Part model, mm, in its own coordinate system. A direction names the side the tool comes from. Round coordinates to 2 decimals unless told otherwise and drop trailing zeros. Loops run counter-clockwise (first coordinate to the right, second up) from the corner with the lowest first, then second, coordinate; pieces in that order, holes last.
Solid Edge part; units mm, degrees
sketch "Sketch1" plane through (0, 0, 0) normal (0, -1, 0) x (1, 0, 0)
  line L0 (-51.028, 6) -> (118.972, 6)
  line L1 (118.972, 6) -> (118.972, -6)
  line L2 (118.972, -6) -> (-51.028, -6)
  line L3 (-51.028, -6) -> (-51.028, 6)
extrude "Protrusion1" add sketch "Sketch1" against normal blind 200
sketch "Sketch2" plane through (33.972, 100, 6) normal (0, 0, 1) x (0, 1, 0)
  line L0 (-100, -85) -> (100, 0)
extrude "ExtrudedCutout_3" cut sketch "Sketch2" against normal blind 139.4118 material side at (76.518, 100.0196, 6)
sketch "Sketch3" plane through (33.972, 0, 0) normal (0, -1, 0) x (1, 0, 0)
  line L0 (-73.94, 3) -> (-73.94, -3)
  line L1 (-73.94, -3) -> (-78.94, 0)
  line L2 (-78.94, 0) -> (-73.94, 3)
extrude "ExtrudedCutout_4" cut sketch "Sketch3" against normal blind 2.5
sketch "Sketch4" plane through (-42.468, 2.5, 0) normal (0, -1, 0) x (0.8574929, 0, -0.5144958)
  circle A0 centre (0, 0) radius 1.25
extrude "ExtrudedCutout_5" cut sketch "Sketch4" against normal blind 2.5
chamfer "Chamfer_6" distance 12 angle 45 2 edges at (76.472, 100, 6) (76.472, 100, -6)
chamfer "Chamfer_7" distance 12 angle 45 2 edges at (-15.0474, 200, 6) (-15.0474, 200, -6)
chamfer "Chamfer_8" distance 12 angle 45 2 edges at (-51.028, 94, 6) (-51.028, 94, -6)
sketch "Sketch5" plane through (33.4526, 94, 6) normal (0, 0, 1) x (1, 0, 0)
  line L0 (-55.9653, 75) -> (-55.9653, 85)
  line L1 (-55.9653, 85) -> (-25.9653, 85)
  line L2 (-25.9653, 85) -> (-25.9653, 75)
  line L3 (-25.9653, 75) -> (-55.9653, 75)
extrude "ExtrudedProtrusion_2" add sketch "Sketch5" along normal blind 10
sketch "Sketch6" plane through (-7.5127, 174, 16) normal (0, 0, 1) x (0, -1, 0)
  line L0 (3, 13) -> (3, -13)
  line L1 (3, -13) -> (-3, -13)
  line L2 (-3, -13) -> (-3, 13)
  line L3 (-3, 13) -> (3, 13)
extrude "ExtrudedCutout_6" cut sketch "Sketch6" against normal blind 10
sketch "Sketch7" plane through (-7.5127, 169, 11) normal (0, -1, 0) x (1, 0, 0)
  line L0 (13, 5) -> (-13, 5)
  line L1 (-13, 5) -> (-13, -5)
  line L2 (-13, -5) -> (13, -5)
  line L3 (13, -5) -> (13, 5)
extrude "ExtrudedCutout_7" cut sketch "Sketch7" against normal blind 74.3913
sketch "Sketch8" plane through (-22.5127, 174, 11) normal (-1, 0, 0) x (0, 0, 1)
  circle A0 centre (0, 0.0043) radius 2.5
extrude "ExtrudedProtrusion_3" add sketch "Sketch8" against normal blind 30
sketch "Sketch9" plane through (33.4526, 94, -6) normal (0, 0, -1) x (0, -1, 0)
  line L0 (-75, 25.9653) -> (-75, 55.9653)
  line L1 (-75, 55.9653) -> (-85, 55.9653)
  line L2 (-85, 55.9653) -> (-85, 25.9653)
  line L3 (-85, 25.9653) -> (-75, 25.9653)
extrude "ExtrudedProtrusion_4" add sketch "Sketch9" along normal blind 10
sketch "Sketch10" plane through (-7.5127, 174, -16) normal (0, 0, -1) x (0, -1, 0)
  line L0 (3, 13) -> (3, -13)
  line L1 (3, -13) -> (-3, -13)
  line L2 (-3, -13) -> (-3, 13)
  line L3 (-3, 13) -> (3, 13)
extrude "ExtrudedCutout_8" cut sketch "Sketch10" against normal blind 10
sketch "Sketch11" plane through (-7.5127, 169, -11) normal (0, -1, 0) x (-1, 0, 0)
  line L0 (13, -5) -> (13, 5)
  line L1 (13, 5) -> (-13, 5)
  line L2 (-13, 5) -> (-13, -5)
  line L3 (-13, -5) -> (13, -5)
extrude "ExtrudedCutout_9" cut sketch "Sketch11" against normal blind 63.7018
sketch "Sketch12" plane through (7.4873, 174, -11) normal (1, 0, 0) x (0, -1, 0)
  circle A0 centre (-0.013, 0) radius 2.5
extrude "ExtrudedProtrusion_5" add sketch "Sketch12" against normal blind 30
1) Slice it at A-A, the plane z = 11. Give the cut face in (x, y), then the cut area to 3 significant figures.
Values:
outline: (-22.51, 169) - (-20.51, 169) - (-20.51, 171.5) - (5.49, 171.5) - (5.49, 169) - (7.49, 169) - (7.49, 179) - (5.49, 179) - (5.49, 176.5) - (-20.51, 176.5) - (-20.51, 179) - (-22.51, 179) - close
area: 170 mm2
2) Wall check: line 1 along X through (y, z) = (173.5, -13.5); line 2 along Z through (x, y) = (26, 175); line 3 along X through (y, z) = (3.7, 0). Give the ranges that are in metal, low to high.
Values:
line 1: x = -22.51 to -20.51, 5.49 to 7.49
line 2: z = -6 to 6
line 3: x = -45.03 to -43.72, -41.22 to 110.88
3) Tool access for faces 1 (the face through (7.487, 174, 11)), 2 (the face through (-41, 2.5, 0)), 3 (the face through (-22.513, 174, -11)), 4 (the face through (5.487, 172, -13)), 5 (the face through (-22.513, 174, 11)): list every direction of +Z, -Z, +X, -X, +Y, -Y with a clear straight run to the whole face (end or side of a thin tool).
Values:
face 1: +Z, +X, +Y, -Y
face 2: -Y
face 3: -Z, -X, +Y, -Y
face 4: none
face 5: +Z, -X, +Y, -Y
4) Slice it at D-D, the plane x = 70. Give the cut face in (y, z), then the cut area to 3 significant figures.
Values:
outline: (0, -6) - (84.55, -6) - (99.9, 0.01) - (84.58, 6) - (0, 6) - close
area: 1,110 mm2
5) Slice it at C-C, the plane y = 96. Give the cut face in (x, z), then the cut area to 3 significant figures.
Values:
outline: (-45.03, 0) - (-39.03, -6) - (65.13, -6) - (71.66, 0.01) - (65.15, 6) - (-39.03, 6) - close
area: 1,330 mm2
6) Drop flat-ended pins along their axis: pin 1 Ø10 at (y, z) = (39, -3.5) entering from +X; pin 2 Ø8 at (y, z) = (172.5, 12) entering from +X; pin 3 Ø8 at (y, z) = (172.5, 13.5) entering from -X. Give the stop position or say it passes through.
Values:
pin 1: stops at x = 97.4
pin 2: stops at x = 7.49
pin 3: stops at x = -22.51
7) Mould opens along X. For faces 6 (the face through (-42.07, 95.64, -2.96)), 7 (the face through (69.09, 94.49, -2.95)), 8 (the face through (35, 0, 0)), 9 (the face through (-7.695, 171.786, 12.154)) say: released by +X, released by -X, zero draft, split by the parting line, or undercut.
Values:
face 6: released by -X
face 7: released by +X
face 8: zero draft
face 9: undercut
8) Slice it at B-B, the plane x = -28.5. Give the cut face in (y, z), then the cut area to 3 significant figures.
Values:
outline: (0, -6) - (188, -6) - (194, 0) - (188, 6) - (0, 6) - close
area: 2,290 mm2
